from build123d import *

# Parameters (mm, degrees)
F0_R     = 1.778
F1_DEPTH = 3.4
F4_DEPTH = 25


with BuildPart() as f1:
    # F0 (on Top) → F1 (new body)
    with BuildSketch(Plane.XY):
        Polygon((50, 10.261858), (0, 10.261858), (-10, 10.261858), (-10, -11.191153), (50, -11.191153), (50, 0), align=None)
        with Locations((-1.3, -5)):
            Circle(F0_R, mode=Mode.SUBTRACT)
        with BuildLine():
            ThreePointArc((8, 0), (12, 4), (16, 0))
            ThreePointArc((16, 0), (14.70562, -2.946119), (11.66019, -3.98554))
            ThreePointArc((11.66019, -3.98554), (11.896688, -4.468462), (11.978, -5))
            ThreePointArc((11.978, -5), (9.125181, -6.41635), (9.721478, -3.287604))
            ThreePointArc((9.721478, -3.287604), (8.456408, -1.855521), (8, 0))
        make_face(mode=Mode.SUBTRACT)
        with Locations((-5, 0)):
            Circle(F0_R, mode=Mode.SUBTRACT)
        with BuildLine():
            ThreePointArc((34, 0), (38, 4), (42, 0))
            ThreePointArc((42, 0), (38, -4), (34, 0))
        make_face(mode=Mode.SUBTRACT)
    extrude(amount=F1_DEPTH)

    # F3 (on face) → F4 (join)
    with BuildSketch(Plane.XY.offset(3.4)):
        Polygon((50, 0), (0, 0), (0, 10.178791), (-2, 10.178791), (-2, -2), (50, -2), align=None)
    extrude(amount=F4_DEPTH)


solid = f1.part
Input: part model. Units: mm. Frame: model coordinates. A direction names the side the tool comes from. Round coordinates to 2 decimals unless told otherwise and drop trailing zeros. Loops run counter-clockwise (first coordinate to the right, second up) from the corner with the lowest first, then second, coordinate; pieces in that order, holes last. Notation, with made-up numbers: M -2,74 L 13,74 A20 ccw 13,103 Z; hole C -34,12 d1. An arc over 180 degrees is marked long. Answer as CSV lines item,"result". Start each with the question number.
(1) Line query: line 1 (X direction, y = 0.5, z = 3); line 2 (Y direction, x = -1.3, z = 1.7); line 3 (Y direction, x = -5, z = 1.05). Output: solid intervals per line, ascending. Write a range as [from, to].
(2) Reachability of faces 1 (the flat face through (20, 0, 0)), 2 (the flat face through (25, 0, 16)), 3 (the flat face through (-2, 4, 16)), 4 (the flat face through (-10, 0, 2)), 5 (the cylindrical face through (34.8, 2.4, 1.7)) from +Z, -Z, +X, -X, +Y, -Y: full face, straight path, thin tool, end or side. Return the list, or none.
(3) Section C-C, the plane x = 17.5. Output: boundary loops of the cut face in (y, z).
(4) Section B-B, the plane y = 2.75. Output: boundary loops of the cut face in (x, z), plus the area to 3 significant figures.
(5) Draft query along Y for faces 6 (the flat face through (24, -2, 16)), 7 (the cylindrical face through (-1.531, -3.237, 1.676)), 8 (the flat face through (-1, 10.179, 16)). Return one class per face: released by +Y, released by -Y, zero draft, split by the parting line, or undercut.
(6) First-contact query: pin 1 (5 mm diameter, centred on x = 17, y = 7.5, fed in from -Z); pin 2 (6 mm diameter, centred on y = 6, z = 12.5, fed in from -X); pin 3 (2 mm diameter, centred on x = 12.5, z = 24.5, fed in from -Y); pin 4 (3 mm diameter, centred on x = 10.2, y = -5, fed in from -Z). Flat tips, straight axial feed; report the tip coordinate or a pass-through.
(7) Section D-D, the plane z = 4. Output: boundary loops of the cut face in (x, y), plus the area to 3 significant figures.
(8) Section A-A, the plane x = -5. Output: boundary loops of the cut face in (y, z).
Values found:
1,line 1,"x = [-10, -6.71], [-3.29, 8.03], [15.97, 34.03], [41.97, 50]"
1,line 2,"y = [-11.19, -6.78], [-3.22, 10.26]"
1,line 3,"y = [-11.19, -1.78], [1.78, 10.26]"
2,face 1,"-Z, +X, -X, +Y, -Y"
2,face 2,"+Z, +X, +Y"
2,face 3,"+Z, -X, +Y, -Y"
2,face 4,"+Z, -Z, -X, +Y, -Y"
2,face 5,"-Z"
3,outline,"M -11.19,0 L 10.26,0 L 10.26,3.4 L 0,3.4 L 0,28.4 L -2,28.4 L -2,3.4 L -11.19,3.4 Z"
4,outline,"M -10,0 L 9.1,0 L 9.1,3.4 L 0,3.4 L 0,28.4 L -2,28.4 L -2,3.4 L -10,3.4 Z; M 14.9,0 L 35.1,0 L 35.1,3.4 L 14.9,3.4 Z; M 40.9,0 L 50,0 L 50,3.4 L 40.9,3.4 Z"
4,area,"214 mm²"
5,face 6,"released by -Y"
5,face 7,"undercut"
5,face 8,"released by +Y"
6,pin 1,"stops at z = 0"
6,pin 2,"stops at x = -2"
6,pin 3,"stops at y = -2"
6,pin 4,"passes through"
7,outline,"M -2,-2 L 50,-2 L 50,0 L 0,0 L 0,10.18 L -2,10.18 Z"
7,area,"124 mm²"
8,outline,"M -11.19,0 L -1.78,0 L -1.78,3.4 L -11.19,3.4 Z; M 1.78,0 L 10.26,0 L 10.26,3.4 L 1.78,3.4 Z"
